Can you work these out from the model? Positions are in its coordinate system, mm. Face numbers are marked on the shaded views. A direction names the side the tool comes from. Round coordinates to 2 decimals unless told otherwise and drop trailing zeros. Loops run counter-clockwise (first coordinate to the right, second up) from the corner with the lowest first, then second, coordinate; pieces in that order, holes last. Notation, with made-up numbers: M 37.25,52.25 L 66.25,52.25 A7 ccw 66.25,64.25 Z; hole C 58,62.5 d3. An arc over 180 degrees is marked long. Use a Markdown table: item, result. Add a question column.
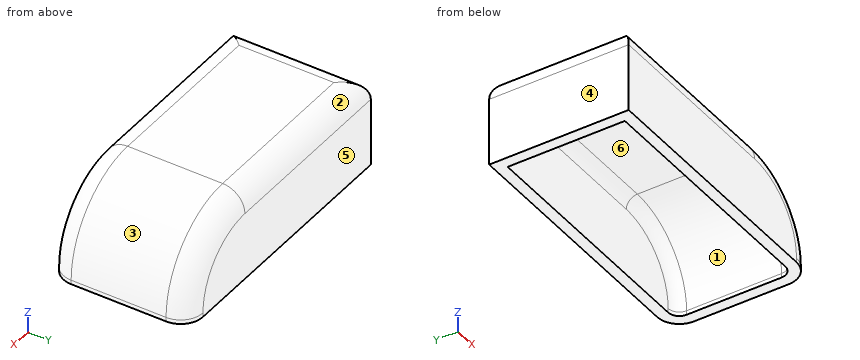
```python
from build123d import *

# Parameters (mm, degrees)
F0_W     = 63.317589
F0_H     = 31.814769
F1_DEPTH = 20.574
F2_R     = 19.622728
F3_R     = 5.08
F4_T     = -2.54


with BuildPart() as f1:
    # F0 (on Top) → F1 (new body)
    with BuildSketch(Plane.XY):
        with Locations((-31.658794, -15.907384)):
            Rectangle(F0_W, F0_H)
    extrude(amount=F1_DEPTH)

    # F2
    f2_edges = [f1.edges().sort_by_distance(p)[0] for p in [
        (0, -15.907384, 20.574),
    ]]
    fillet(f2_edges, radius=F2_R)

    # F3
    f3_edges = [f1.edges().sort_by_distance(p)[0] for p in [
        (-41.470159, -31.814769, 20.574),
        (-41.470159, 0, 20.574),
        (-63.317589, -15.907384, 20.574),
    ]]
    fillet(f3_edges, radius=F3_R)

    # F4
    f4_openings = [f1.faces().sort_by_distance(p)[0] for p in [
        (-31.827557, -15.907384, 0),
    ]]
    offset(amount=F4_T, openings=f4_openings)


solid = f1.part
```
(1) On a 3-axis mill with a long thin cutter (end or side, diameter ignored), from which of +Z, -Z, +X, -X, +Y, -Y can I reach the whole of each face in a straight line? I mean the marked faces 5 and 6. Say none if no direction works.
(2) Thinking about a two-plate mould opening in X: for the marked faces 1, 2, 3 and 4, which applies, released by +X, released by -X, zero draft, split by the parting line, or undercut?
(3) If I drill on probe 1 along Y at (x, z) = (-40, 8.5); probe 2 along Y at (x, z) = (-58, 15.75); probe 3 along Z at (x, y) = (-24, -27), over which ranges is the centre line in solid material (lowest first)? Write a range as [from, to].
(4) I'm going to push flat-ended pins straight in: pin 1 (6 mm diameter, centred on y = -15, z = 11, fed in from +X); pin 2 (3 mm diameter, centred on y = -4.5, z = 14.5, fed in from +X); pin 3 (6 mm diameter, centred on y = -27.5, z = 4.5, fed in from +X). Where does each tip first touch, or does it pass through?
(5) Suppose I cut it at B-B on y = -9. List the corners of the cut face in (x, z) for me, and give its area (3 significant figures).
(6) Suppose I cut it at A-A on x = -41. List the corners of the cut face in (y, z) for me.
Results below:
| question | item | result |
|---|---|---|
| 1 | face 5 | +Z, -Z, +X, -X, +Y |
| 1 | face 6 | -Z |
| 2 | face 1 | undercut |
| 2 | face 2 | zero draft |
| 2 | face 3 | released by +X |
| 2 | face 4 | released by -X |
| 3 | probe 1 | y = [-31.81, -29.27], [-2.54, 0] |
| 3 | probe 2 | y = [-31.81, -29.26], [-2.55, -0.01] |
| 3 | probe 3 | z = [18.02, 20.57] |
| 4 | pin 1 | stops at x = -1.31 |
| 4 | pin 2 | stops at x = -4.16 |
| 4 | pin 3 | stops at x = -0.01 |
| 5 | outline | M -63.32,0 L -60.78,0 L -60.78,15.49 A2.54 cw -58.24,18.03 L -19.62,18.03 A17.08 cw -2.54,0.95 L -2.54,0 L 0,0 L 0,0.95 A19.62 ccw -19.62,20.57 L -58.24,20.57 A5.08 ccw -63.32,15.49 Z |
| 5 | area | 228 mm² |
| 6 | outline | M -31.81,0 L -29.27,0 L -29.27,15.49 A2.54 cw -26.73,18.03 L -5.08,18.03 A2.54 cw -2.54,15.49 L -2.54,0 L 0,0 L 0,15.49 A5.08 ccw -5.08,20.57 L -26.73,20.57 A5.08 ccw -31.81,15.49 Z |
